Here's how the part is built. I have some questions about the finished solid (model axes, mm). A direction names the side the tool comes from. Give positions to 0.01 mm unless a question says otherwise; leave off trailing zeros. Order: outer loops, then holes, each group sorted by start corner. A loop starts at its lowest first (then second) coordinate and runs counter-clockwise, first axis right, second up.
Autodesk Fusion 360 part; units mm, degrees
sketch "スケッチ1" plane through (0, 0, 0) normal (0, 0, 1) x (1, 0, 0)
  line L0 (-500, 0) -> (500, 0)
  line L1 (500, 0) -> (500, -1000)
  line L2 (-500, -1000) -> (-500, 0)
  line L3 (-400, -100) -> (362.4762, -100)
  line L4 (400, -137.5238) -> (400, -500)
  line L5 (400, -500) -> (-362.4762, -500)
  line L6 (-400, -462.4762) -> (-400, -100)
  line L7 (-362.4762, -600) -> (400, -600)
  line L8 (400, -600) -> (400, -962.4762)
  line L9 (400, -1000) -> (362.4762, -1000)
  line L10 (-400, -1000) -> (-400, -637.5238)
  line L11 (-400, -462.4762) -> (362.4762, -100)
  line L12 (400, -137.5238) -> (-362.4762, -500)
  line L13 (-362.4762, -600) -> (400, -962.4762)
  line L14 (362.4762, -1000) -> (-400, -637.5238)
  line L15 (500, -1000) -> (362.4762, -1000)
  line L16 (-400, -1000) -> (-500, -1000)
  line L17 (-400, -462.4762) -> (-400, -500) construction
  line L18 (-400, -500) -> (-362.4762, -500) construction
  line L19 (-362.4762, -600) -> (-400, -600) construction
  line L20 (-400, -600) -> (-400, -637.5238) construction
  line L21 (362.4762, -100) -> (400, -100) construction
  line L22 (400, -100) -> (400, -137.5238) construction
  line L23 (400, -962.4762) -> (400, -1000) construction
  line L24 (-400, -1000) -> (362.4762, -1000) construction
  dimension "d5" = 400
  dimension "d6" = 800
  dimension "d7" = 100
  dimension "d8" = 100
  dimension "d9" = 100
  dimension "d10" = 100
  dimension "d11" = 400
  dimension "d12" = 50
  dimension "d13" = 50
extrude "押し出し1" add sketch "スケッチ1" along normal blind 100
fillet "フィレット1" radius 50 1 edges at (-500, -500, 100)
fillet "フィレット2" radius 50 1 edges at (-400, -281.2381, 100)
fillet "フィレット3" radius 50 1 edges at (-400, -818.7619, 100)
fillet "フィレット4" radius 50 3 edges at (400, -318.7619, 100) (400, -781.2381, 100) (500, -500, 100)
fillet "フィレット5" radius 50 6 edges at (-500, -500, 0) (-400, -818.7619, 0) (-400, -281.2381, 0) (400, -318.7619, 0) (400, -781.2381, 0) (500, -500, 0)
Q1. I'm going to push flat-ended pins straight in: P1, Ø6, axis at y = -206.5, z = 74.5, coming from the +X side; P2, Ø2, axis at y = -149, z = 62, coming from the +X side; P3, Ø5, axis at y = -684.5, z = 18, coming from the -X side. Where does each tip first touch, or does it pass through?
Filled sheet:
P1: stops at x = 495.15
P2: stops at x = 498.78
P3: stops at x = -490.38
Q2. Thinking about a two-plate mould opening in Y: for faces 1 (the face through (-49, -100, 49)), 2 (the face through (-7, 0, 49)), 3 (the face through (415.03, -309.58, 85.74)), 4 (the face through (-414.26, -804.18, 15.03)), which applies, released by +Y, released by -Y, zero draft, split by the parting line, or undercut?
Filled sheet:
face 1: undercut
face 2: released by +Y
face 3: undercut
face 4: zero draft
Q3. If we section it at B-B on x = 387.5: List the corners of the cut face in (y, z) for me, plus the area to 3 significant figures.
Filled sheet:
outline: (-1000, 0) - (-956.53, 0) - (-956.53, 100) - (-1000, 100) - close; (-600, 0) - (-500, 0) - (-500, 100) - (-600, 100) - close; (-143.47, 0) - (0, 0) - (0, 100) - (-143.47, 100) - close
area: 28,700 mm2
Q4. For faces 5 (the face through (-415.03, -804.18, 85.74)), 6 (the face through (414.26, -795.82, 15.03)), 7 (the face through (-484.97, -493, 14.26)), which set-ups out of +Z, -Z, +X, -X, +Y, -Y let a thin tool reach every point of the face, with its end or its side?
Filled sheet:
face 5: +Z, -Y
face 6: -Z
face 7: -Z, -X, +Y, -Y
Q5. I need wall thicknesses on L1, parallel to X at y = -834.5, z = 42.5; L2, parallel to X at y = -434, z = 34; L3, parallel to Y at x = 25.5, z = 20. Which ranges of each line are inside material? Lowest first, please.
Filled sheet:
L1: x = -499.44 to -400.56, 14.34 to 130.8, 400.56 to 499.44
L2: x = -497.37 to -402.63, -340.1 to -223.64, 402.63 to 497.37
L3: y = -839.8 to -784.44, -600 to -500, -315.56 to -260.2, -100 to 0
Q6. If we section it at D-D on x = 36: List the corners of the cut face in (y, z) for me.
Filled sheet:
outline: (-844.8, 0) - (-789.43, 0) - (-789.43, 100) - (-844.8, 100) - close; (-600, 0) - (-500, 0) - (-500, 100) - (-600, 100) - close; (-310.57, 0) - (-255.2, 0) - (-255.2, 100) - (-310.57, 100) - close; (-100, 0) - (0, 0) - (0, 100) - (-100, 100) - close
Q7. If we section it at C-C on z = 83: List the corners of the cut face in (x, y) for me, plus the area to 3 significant figures.
Filled sheet:
outline: (-487.56, -1000) - (-412.43, -1000) - (-412.43, -631.61) - (362.48, -1000) - (487.57, -1000) - (487.57, 0) - (-487.56, 0) - close; hole (-412.43, -468.39) - (362.48, -100) - (-412.43, -100) - close; hole (-362.48, -600) - (412.43, -968.39) - (412.43, -600) - close; hole (-362.48, -500) - (412.43, -500) - (412.43, -131.61) - close
area: 404,000 mm2
Q8. If we section it at A-A on y = -207: Give the number of separate pieces and of enclosed holes in the cut face, plus the area to 3 significant figures.
Filled sheet:
separate pieces: 3
enclosed holes: 0
area: 27,400 mm2
